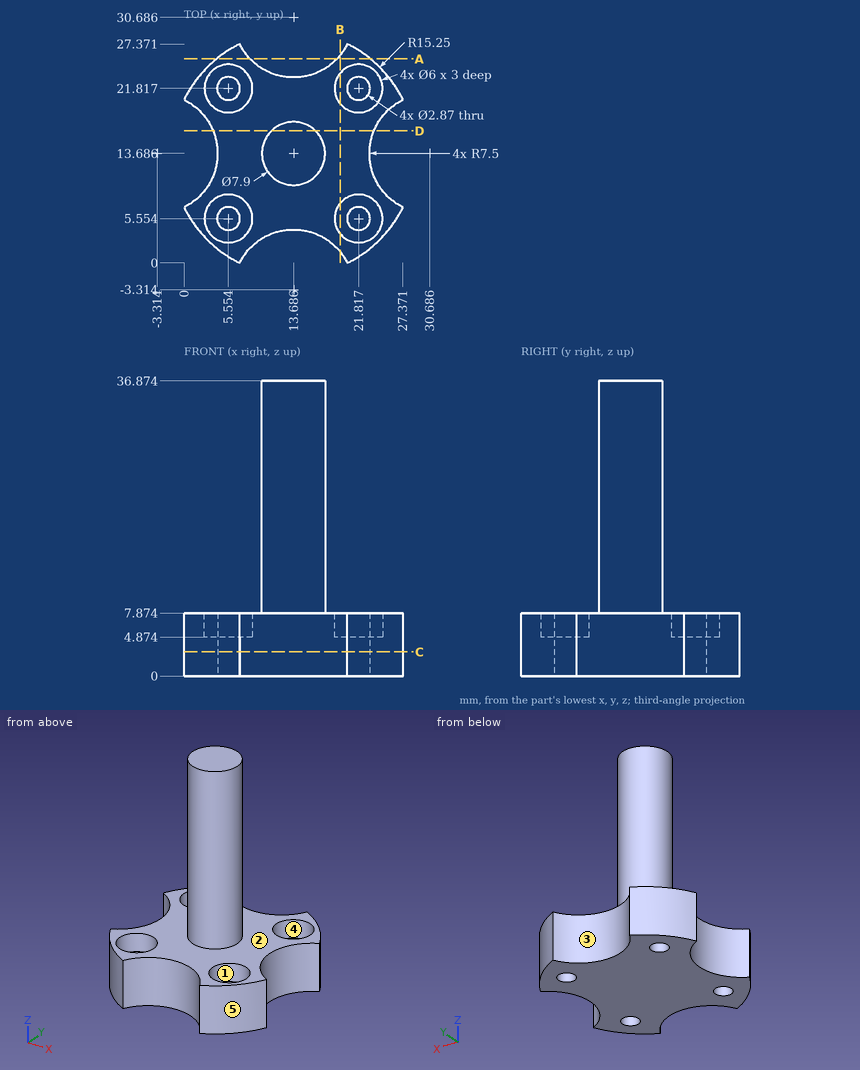
The drawing under review shows one solid part. Ordinate dimensions are in mm from its lowest x, y, z. A direction names the side the tool comes from. Round coordinates to 2 decimals unless told otherwise and drop trailing zeros. Loops run counter-clockwise (first coordinate to the right, second up) from the corner with the lowest first, then second, coordinate; pieces in that order, holes last.
Item 1: Take a section at A-A (y = 25.5). Write out the cut boundary in (x, z).
Determined:
outline: (4.04, 0) - (8.27, 0) - (8.27, 7.87) - (4.04, 7.87) - close; (19.1, 0) - (23.33, 0) - (23.33, 7.87) - (19.1, 7.87) - close
Item 2: Mouldability with a two-part tool opening along Y and no side actions: class the marked faces 1, 2 and 3 as released by +Y, released by -Y, zero draft, split by the parting line, or undercut.
Determined:
face 1: undercut
face 2: zero draft
face 3: released by +Y
Item 3: Take a section at D-D (y = 16.5). Write out the cut boundary in (x, z).
Determined:
outline: (3.64, 0) - (23.73, 0) - (23.73, 7.87) - (16.46, 7.87) - (16.46, 36.87) - (10.91, 36.87) - (10.91, 7.87) - (3.64, 7.87) - close
Item 4: For the marked faces 4 and 5, list the 3-axis set-ups (+Z, -Z, +X, -X, +Y, -Y) from which the entire face can be reached by the end or side of a thin tool; tool diameter is ignored.
Determined:
face 4: +Z
face 5: +Z, -Z, +X, -Y
Item 5: Take a section at B-B (x = 19.5). Write out the cut boundary in (y, z).
Determined:
outline: (1.42, 0) - (25.95, 0) - (25.95, 7.87) - (23.72, 7.87) - (23.72, 4.87) - (19.91, 4.87) - (19.91, 7.87) - (7.46, 7.87) - (7.46, 4.87) - (3.65, 4.87) - (3.65, 7.87) - (1.42, 7.87) - close
Item 6: Take a section at C-C (z = 3). Give the number of separate pieces and of enclosed holes in the cut face, then the cut area to 3 significant figures.
Determined:
separate pieces: 1
enclosed holes: 4
area: 487 mm2
Item 7: For line 1 (Z direction, x = 26.25, y = 21.25); line 2 (X direction, y = 2, z = 5.5) (1 decimal); line 3 (Z direction, x = 6.5, y = 7.25), list the stretches that pass through material, from the lowest coordinate up.
Determined:
line 1: z = 0 to 7.87
line 2: x = 3.9 to 8.4, 19 to 23.5
line 3: z = 0 to 4.87
Item 8: Clearance check with flat-ended pins moving along their axes: pin 1 Ø6.5 at (x, y) = (5, 5.5) entering from +Z; pin 2 Ø1.7 at (x, y) = (5.55, 21.82) entering from +Z; pin 3 Ø3 at (y, z) = (10.5, 26.5) entering from -X; pin 4 Ø3 at (x, y) = (21.5, 21.5) entering from +Z. State where each tip first meets the part, or that it passes through.
Determined:
pin 1: stops at z = 7.87
pin 2: passes through
pin 3: stops at x = 10.11
pin 4: stops at z = 4.87
